Geometry check sheet. Reference: drawing and pictorial views, mm from the part's lowest x, y, z. Round coordinates to 2 decimals unless told otherwise and drop trailing zeros. Return JSON: item names as keys, results as strings.
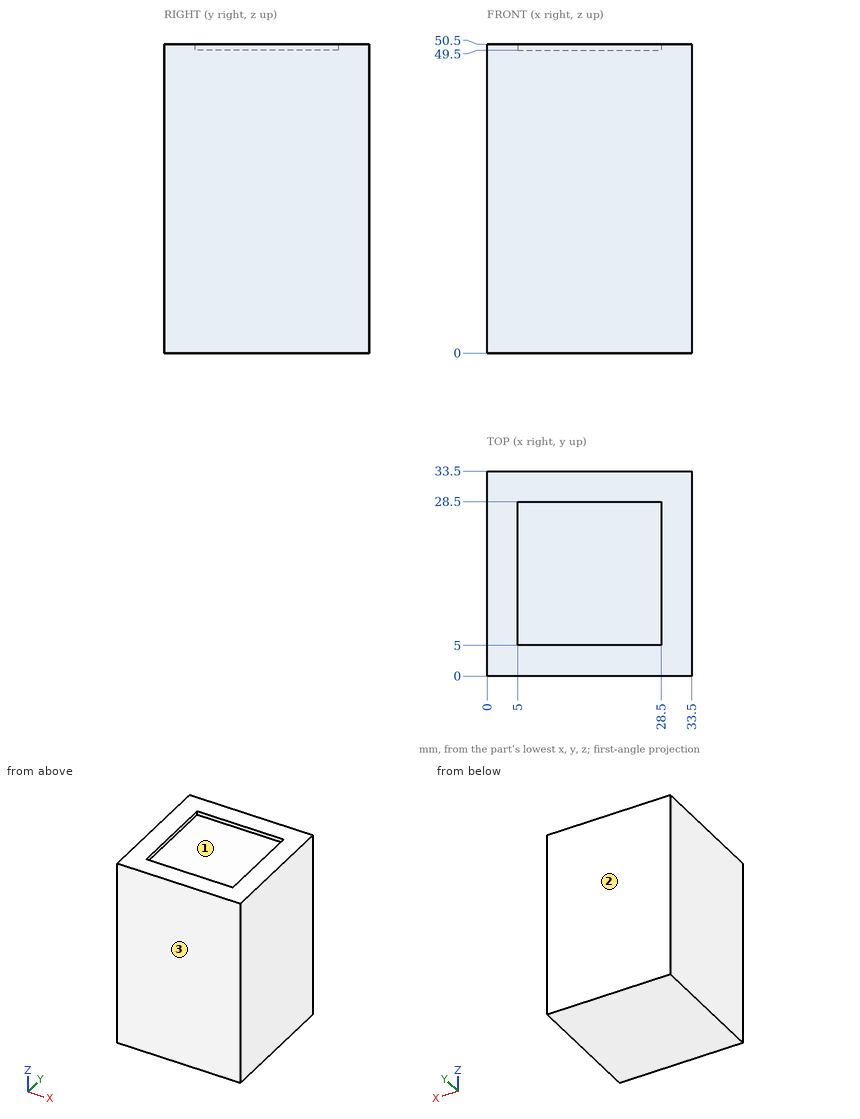
(1) Release check for a two-part mould opening along Y. For the marked faces 1, 2 and 3 record: pulls with the +Y half, pulls with the -Y half, needs draft (parallel to the pull), parting line crosses it, or undercut.
Response values:
{"face 1": "undercut", "face 2": "pulls with the +Y half", "face 3": "pulls with the -Y half"}
(2) Material ranges on line 1 along Z through (x, y) = (10.5, 21.5), recorded low to high. Write a range as [from, to].
Response values:
{"line 1": "z = [0, 49.5]"}
(3) Gauge pin test, flat ends, axial feed: pin 1 (4 mm diameter, centred on y = 11.5, z = 19.5, fed in from -X); pin 2 (6 mm diameter, centred on x = 9.5, y = 15, fed in from +Z). Record the tip position at first contact, or that the pin passes through.
Response values:
{"pin 1": "stops at x = 0", "pin 2": "stops at z = 49.5"}
